For this review, take the finished solid that the model builds, in its own axes (mm). Face numbers are marked on the shaded views. Round coordinates to 2 decimals unless told otherwise and drop trailing zeros. Order: outer loops, then holes, each group sorted by start corner. A loop starts at its lowest first (then second) coordinate and runs counter-clockwise, first axis right, second up. Notation, with made-up numbers: M -14.75,48.25 L -2.75,48.25 A23 ccw -2.75,75.25 Z; hole C 44.25,13.5 d4. An arc over 180 degrees is marked long. Put each result on its own line as item: value.
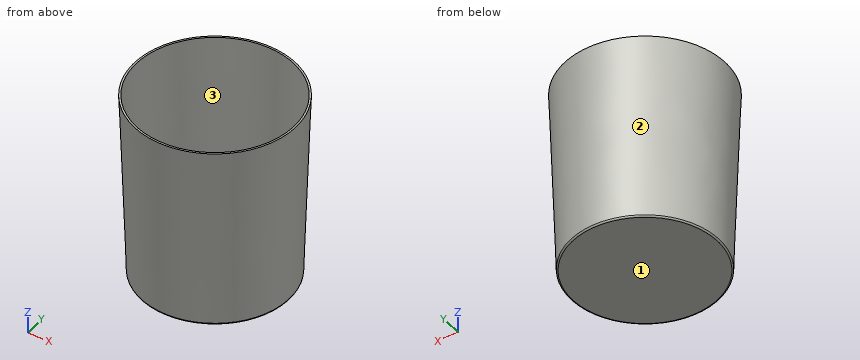
from build123d import *

# Parameters (mm, degrees)
F0_R     = 100
F1_DEPTH = 250
F1_TAPER = -2
F2_T     = -2.5
F3_R     = 2


with BuildPart() as f1:
    # F0 (on Top) → F1 (new body)
    with BuildSketch(Plane.XY):
        Circle(F0_R)
    extrude(amount=F1_DEPTH, taper=F1_TAPER)

    # F2
    f2_openings = [f1.faces().sort_by_distance(p)[0] for p in [
        (0, 0, 250),
    ]]
    offset(amount=F2_T, openings=f2_openings, kind=Kind.INTERSECTION)

    # F3
    f3_edges = [f1.edges().sort_by_distance(p)[0] for p in [
        (-100, 0, 0),
        (-97.585778, 0, 2.5),
    ]]
    fillet(f3_edges, radius=F3_R)


solid = f1.part
(1) Draft analysis for pull direction X (two halves, no side actions). For the marked faces 1, 2 and 3, state which applies: released by +X, released by -X, zero draft, split by the parting line, or undercut.
A:
face 1: zero draft
face 2: split by the parting line
face 3: undercut
(2) Add section B-B on z = 199. Give the boundary of the cut face in (x, y).
A:
outline: C 0,0 d213.9; hole C 0,0 d208.9
(3) Add section C-C on z = 32.5. Give the boundary of the cut face in (x, y).
A:
outline: C 0,0 d202.27; hole C 0,0 d197.27
(4) Insertion check: pin 1 Ø1.5 at (x, y) = (12.5, 57.5) entering from +Z; pin 2 Ø10 at (x, z) = (-32.5, 96.5) entering from -Y; pin 3 Ø3 at (x, y) = (-80.5, -52) entering from +Z (3 decimals). Each pin has a flat end and moves straight along its axis. Give the tip position at first contact, or say it passes through.
A:
pin 1: stops at z = 2.5
pin 2: stops at y = -99.66
pin 3: stops at z = 3.415
(5) To check wall thickness, follow L1, parallel to Z at x = 62.5, y = 48.5; L2, parallel to Y at x = -92.5, z = 187; L3, parallel to Y at x = 64, z = 204.5. State the ranges of each line that lie inside material, in increasing order.
A:
L1: z = 0 to 2.5
L2: y = -52.84 to -47.6, 47.6 to 52.84
L3: y = -85.93 to -82.79, 82.79 to 85.93
(6) Add section A-A on x = 0. Give the boundary of the cut face in (y, z).
A:
outline: M -108.73,250 L -100.07,1.93 A2 ccw -98.07,0 L 98.07,0 A2 ccw 100.07,1.93 L 108.73,250 L 106.23,250 L 97.65,4.43 A2 cw 95.65,2.5 L -95.65,2.5 A2 cw -97.65,4.43 L -106.23,250 Z
